For this review, take the finished solid that the model builds, in its own axes (mm). Face numbers are marked on the shaded views. A direction names the side the tool comes from. Round coordinates to 2 decimals unless told otherwise and drop trailing zeros. Loops run counter-clockwise (first coordinate to the right, second up) from the corner with the lowest first, then second, coordinate; pieces in that order, holes last.
```python
from build123d import *

# Parameters (mm, degrees)
SKETCH_1_R          = 8.5
EXTRUDE_1_DEPTH     = 43
SKETCH_2_R          = 5
EXTRUDE_2_DEPTH     = 3.5
SKETCH_3_R          = 2.5
EXTRUDE_3_DEPTH     = 9
SKETCH_4_R          = 1.5
CUT_EXTRUDE_1_DEPTH = 10
SKETCH_5_R          = 4.5
SKETCH_5_R_2        = 2.5
EXTRUDE_4_DEPTH     = 2


with BuildPart() as part:
    # Sketch 1 → Extrude 1 (new body)
    with BuildSketch(Plane(origin=(0, 0, 0), x_dir=(1, 0, 0), z_dir=(0, 1, 0))):
        with Locations(Location((0, 0, 0), (0, 0, 270))):
            Circle(SKETCH_1_R)
    extrude(amount=EXTRUDE_1_DEPTH)



with BuildPart() as body_2:
    # Sketch 2 → Extrude 2 (new, symmetric)
    with BuildSketch(Plane.XY):
        with Locations((0, 55)):
            Circle(SKETCH_2_R)
    extrude(amount=EXTRUDE_2_DEPTH, both=True)


with BuildPart() as part_1:
    add(part.part)

    add(body_2.part)  # Extrude 3 merges body 2
    # Sketch 3 → Extrude 3 (add)
    with BuildSketch(Plane(origin=(0, 43, 0), x_dir=(1, 0, 0), z_dir=(0, 1, 0))):
        with Locations(Location((0, 0, 0), (0, 0, 90))):
            Circle(SKETCH_3_R)
    extrude(amount=EXTRUDE_3_DEPTH)

    # Sketch 4 → Cut-Extrude 1 (cut)
    with BuildSketch(Plane.XY.offset(3.5)):
        with Locations((0, 55)):
            Circle(SKETCH_4_R)
    extrude(amount=-CUT_EXTRUDE_1_DEPTH, mode=Mode.SUBTRACT)

    # Sketch 5 → Extrude 4 (add)
    with BuildSketch(Plane(origin=(0, 43, 0), x_dir=(1, 0, 0), z_dir=(0, 1, 0))):
        with Locations(Location((0, 0, 0), (0, 0, 270))):
            Circle(SKETCH_5_R)
        with Locations(Location((0, 0, 0), (0, 0, 90))):
            Circle(SKETCH_5_R_2, mode=Mode.SUBTRACT)
    extrude(amount=EXTRUDE_4_DEPTH)


solid = part_1.part
```
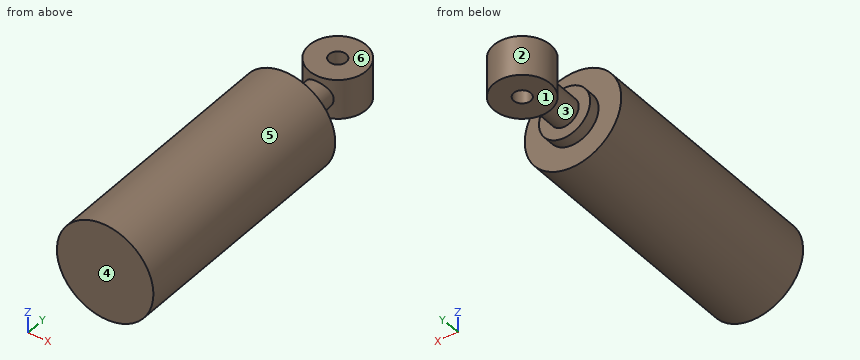
(1) Add section B-B (z = 0). Give the boundary of the cut face in (x, y), plus the area to 3 significant figures.
(2) Insertion check: pin 1 Ø1 at (y, z) = (44, -2) entering from -X; pin 2 Ø10 at (x, z) = (1, 2) entering from +Y; pin 3 Ø8 at (x, y) = (-2, 55.5) entering from -Z; pin 4 Ø8 at (x, y) = (1.5, 57) entering from +Z. Each pin has a flat end and moves straight along its axis. Give the tip position at first contact, or say it passes through.
(3) Add section C-C (x = 5.75). Give the boundary of the cut face in (y, z).
(4) For L1, parallel to Y at x = 0, z = 0.25; L2, parallel to Y at x = -7.5, z = 1.75; L3, parallel to Z at x = 0.25, y = 34, list the stretches that pass through material, from the lowest coordinate up.
(5) Add section A-A (y = 55). Give the boundary of the cut face in (x, z), plus the area to 3 significant figures.
(6) The part is to be moulded in two halves that separate along Y. For the marked faces 1, 2, 3 and 4, say which applies: pulls with the +Y half, pulls with the -Y half, needs draft (parallel to the pull), parting line crosses it, or undercut.
(7) Add section D-D (y = 47). Give the boundary of the cut face in (x, z), plus the area to 3 significant figures.
(8) For the marked faces 5 and 6, list the 3-axis set-ups (+Z, -Z, +X, -X, +Y, -Y) from which the entire face can be reached by the end or side of a thin tool; tool diameter is ignored.
Outcome:
1. outline: (-8.5, 0) - (8.5, 0) - (8.5, 43) - (4.5, 43) - (4.5, 45) - (2.5, 45) - (2.5, 50.67) arc R5 ccw (long way) to (-2.5, 50.67) - (-2.5, 45) - (-4.5, 45) - (-4.5, 43) - (-8.5, 43) - close; hole circle Ø3 at (0, 55)
1. area: 847 mm2
2. pin 1: stops at x = -4.24
2. pin 2: stops at y = 60
2. pin 3: stops at z = -3.5
2. pin 4: stops at z = 3.5
3. outline: (0, -6.26) - (43, -6.26) - (43, 6.26) - (0, 6.26) - close
4. L1: y = 0 to 53.5, 56.5 to 60
4. L2: y = 0 to 43
4. L3: z = -8.5 to 8.5
5. outline: (-5, -3.5) - (-1.5, -3.5) - (-1.5, 3.5) - (-5, 3.5) - close; (1.5, -3.5) - (5, -3.5) - (5, 3.5) - (1.5, 3.5) - close
5. area: 49.0 mm2
6. face 1: needs draft
6. face 2: undercut
6. face 3: undercut
6. face 4: pulls with the -Y half
7. outline: circle Ø5 at (0, 0)
7. area: 19.6 mm2
8. face 5: +Y, -Y
8. face 6: +Z, +X, -X, +Y
